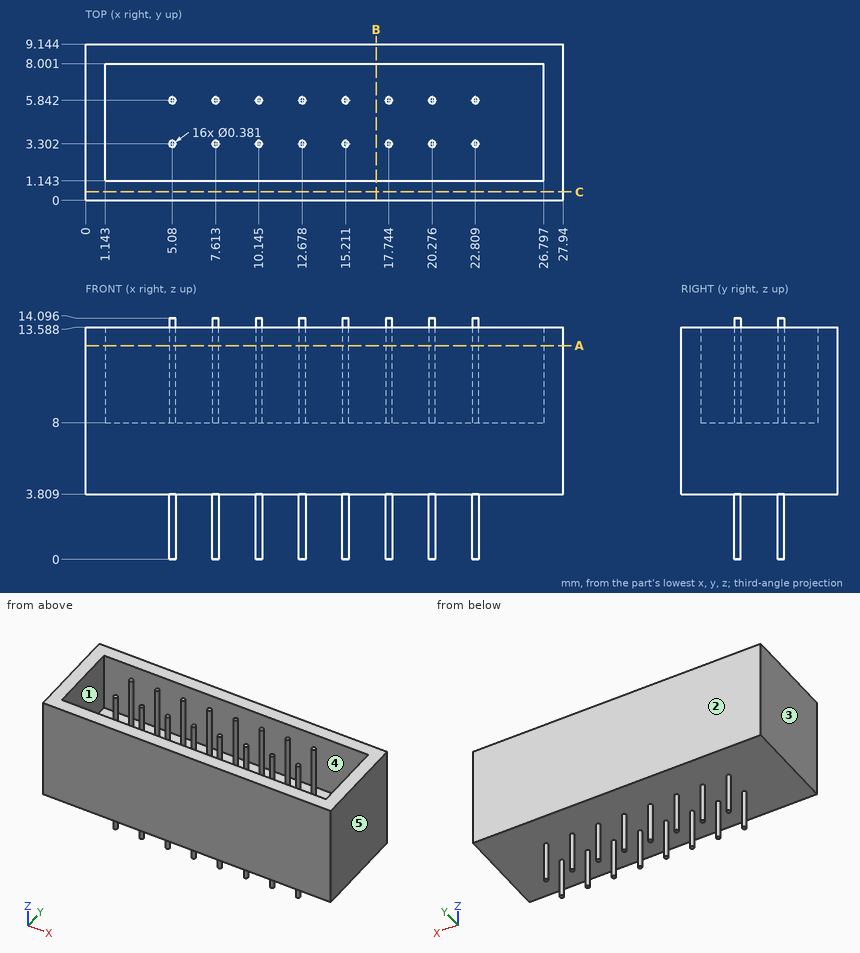
Design review of the part shown in the three views and the two pictorial views. Dimensions are in mm from the part's minimum x, y and z. A direction names the side the tool comes from. Round coordinates to 2 decimals unless told otherwise and drop trailing zeros. Write each loop counter-clockwise with the first axis right and the second up, starting at its lowest first coordinate (ties: lowest second). Pieces come first, ordered by that corner, then holes.
Item 1: Consider section B-B on x = 17. Give the boundary of the cut face in (y, z).
Item 2: Consider section A-A on z = 12.5. Count the separate pieces of the cut face and the enclosed holes in it.
Item 3: Draft analysis for pull direction X (two halves, no side actions). For the marked faces 3, 4 and 5, state which applies: released by +X, released by -X, zero draft, split by the parting line, or undercut.
Item 4: Wall thickness on L1, parallel to Y at x = 8.25, z = 11.25; L2, parallel to X at y = 2.25, z = 12.5; L3, parallel to Z at x = 6.75, y = 7.75: over which ranges is each line inside the solid? List them lowest first.
Item 5: For the marked faces 1 and 2, list the 3-axis set-ups (+Z, -Z, +X, -X, +Y, -Y) from which the entire face can be reached by the end or side of a thin tool; tool diameter is ignored.
Item 6: For pin 1 Ø1 at (x, y) = (4.5, 4) entering from -Z, flat-tipped, find the tip position at first contact; note if it passes through.
Item 7: Consider section C-C on y = 0.5. Give the boundary of the cut face in (x, z).
Check values:
1. outline: (0, 3.81) - (9.14, 3.81) - (9.14, 13.59) - (8, 13.59) - (8, 8) - (1.14, 8) - (1.14, 13.59) - (0, 13.59) - close
2. separate pieces: 17
2. enclosed holes: 1
3. face 3: released by -X
3. face 4: undercut
3. face 5: released by +X
4. L1: y = 0 to 1.14, 8 to 9.14
4. L2: x = 0 to 1.14, 26.8 to 27.94
4. L3: z = 3.81 to 8
5. face 1: +Z
5. face 2: +Z, -Z, +X, -X, +Y
6. pin 1: stops at z = 3.81
7. outline: (0, 3.81) - (27.94, 3.81) - (27.94, 13.59) - (0, 13.59) - close
